For this review, use the dimensioned drawing (mm, ordinates from the lowest corner) and the shaded views. A direction names the side the tool comes from. Coordinates: 2 decimals unless noted, no trailing zeros. Write each loop counter-clockwise with the first axis right and the second up, starting at its lowest first coordinate (ties: lowest second). Pieces come first, ordered by that corner, then holes. Notation, with made-up numbers: (71.5, 18) - (86.5, 18) arc R8 cw to (86.5, 28) - close; hole circle Ø2 at (-33.5, 7). An arc over 180 degrees is marked (long way). Answer as a JSON object with one key per item and string values.
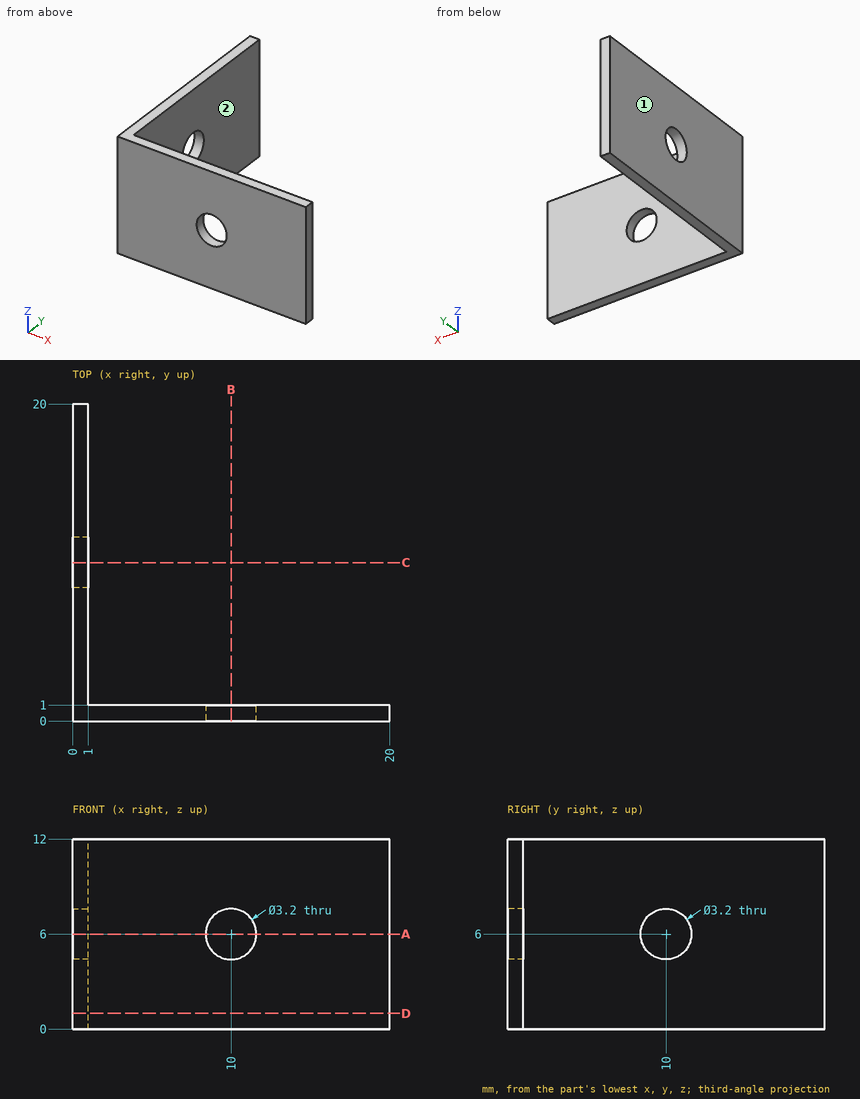
(1) Take a section at A-A, the plane z = 6. Write out the cut boundary in (x, y).
Solved:
{"outline": "(0, 0) - (8.4, 0) - (8.4, 1) - (1, 1) - (1, 8.4) - (0, 8.4) - close; (0, 11.6) - (1, 11.6) - (1, 20) - (0, 20) - close; (11.6, 0) - (20, 0) - (20, 1) - (11.6, 1) - close"}
(2) Take a section at B-B, the plane x = 10. Write out the cut boundary in (y, z), and give its area (3 significant figures).
Solved:
{"outline": "(0, 0) - (1, 0) - (1, 4.4) - (0, 4.4) - close; (0, 7.6) - (1, 7.6) - (1, 12) - (0, 12) - close", "area": "8.80 mm^2"}
(3) For pin 1 (1.5 mm diameter, centred on x = 10.5, z = 9, fed in from +Y); pin 2 (4 mm diameter, centred on y = 11, z = 9, fed in from -X), all flat-tipped, find the tip position at first contact; note any pin that passes through.
Solved:
{"pin 1": "stops at y = 1", "pin 2": "stops at x = 0"}
(4) Tool access review of the marked faces 1 and 2: name each direction out of +Z, -Z, +X, -X, +Y, -Y from which nothing blocks a thin tool from reaching the whole face with its end or side.
Solved:
{"face 1": "+Z, -Z, -X, +Y, -Y", "face 2": "+Z, -Z, +X, +Y"}
(5) Take a section at D-D, the plane z = 1. Write out the cut boundary in (x, y).
Solved:
{"outline": "(0, 0) - (20, 0) - (20, 1) - (1, 1) - (1, 20) - (0, 20) - close"}
(6) To check wall thickness, follow line 1 (Y direction, x = 0.5, z = 6); line 2 (Z direction, x = 10, y = 0.4); line 3 (X direction, y = 13.25, z = 10.25). State the ranges of each line that lie inside material, in increasing order. Write a range as from..to.
Solved:
{"line 1": "y = 0..8.4, 11.6..20", "line 2": "z = 0..4.4, 7.6..12", "line 3": "x = 0..1"}
